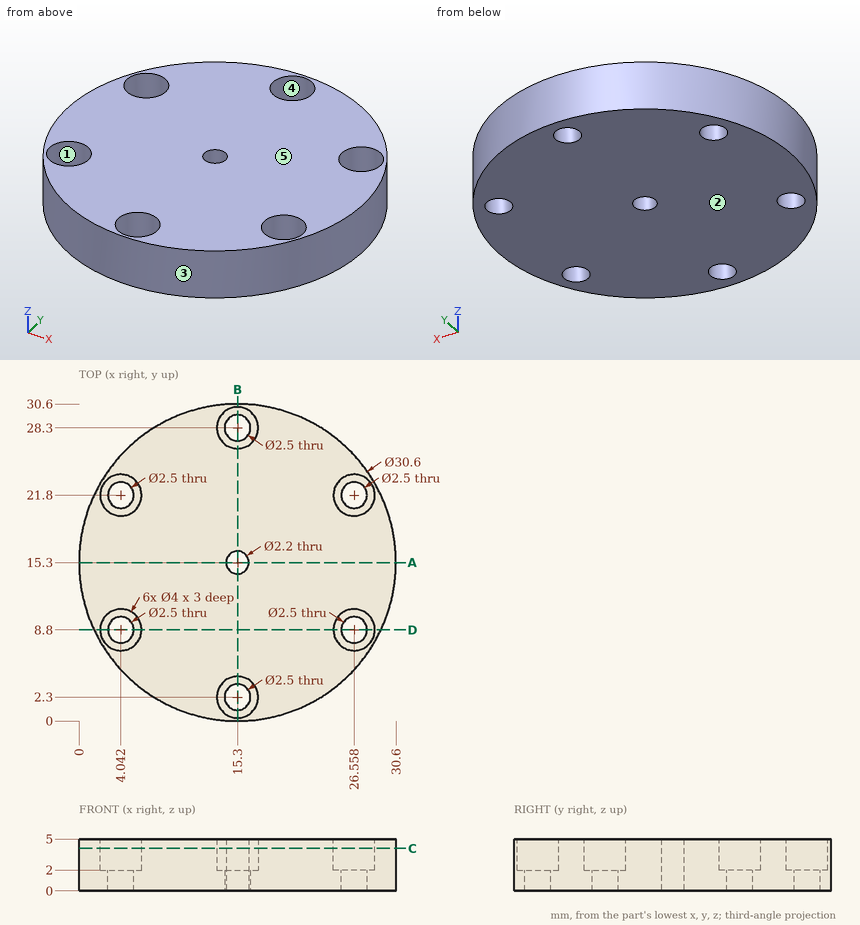
Part print with two shaded views. Sizes in mm from the minimum x, y, z corner. A direction names the side the tool comes from. Round coordinates to 2 decimals unless told otherwise and drop trailing zeros. Loops run counter-clockwise (first coordinate to the right, second up) from the corner with the lowest first, then second, coordinate; pieces in that order, holes last.
Item 1: Saw through at B-B (x = 15.3). List the corners of the cut face in (y, z).
Item 2: Saw through at A-A (y = 15.3). List the corners of the cut face in (x, z), then the cut area to 3 significant figures.
Item 3: Pin check, flat tips, straight feed: P1, Ø2, axis at x = 12, z = 2, coming from the +Y side; P2, Ø2, axis at x = 18, z = 1, coming from the +Y side (1 decimal); P3, Ø3, axis at x = 26.56, y = 8.8, coming from the +Z side. Stop position of each tip, or through.
Item 4: Which spindle directions (+Z, -Z, +X, -X, +Y, -Y) get a long thin tool onto all of the face, cutting with end or side? Do the marked faces 4 and 5. Say none if no direction does.
Item 5: Saw through at C-C (z = 4.1). List the corners of the cut face in (x, y), then the cut area to 3 significant figures.
Item 6: Drill centre lines: line 1 along Y through (x, z) = (15.3, 2.9); line 2 along Y through (x, z) = (15.3, 0.65); line 3 along X through (y, z) = (9.5, 1.15) (1 decimal). Where is each one in solid material? Low to high.
Item 7: Two-plate mould, pull along Y, no slides. Class the marked faces 1, 2 and 3: released by +Y, released by -Y, zero draft, split by the parting line, or undercut.
Item 8: Saw through at D-D (y = 8.8). List the corners of the cut face in (x, z).
Worked answers:
1. outline: (0, 0) - (1.05, 0) - (1.05, 2) - (0.3, 2) - (0.3, 5) - (0, 5) - close; (3.55, 0) - (14.2, 0) - (14.2, 5) - (4.3, 5) - (4.3, 2) - (3.55, 2) - close; (16.4, 0) - (27.05, 0) - (27.05, 2) - (26.3, 2) - (26.3, 5) - (16.4, 5) - close; (29.55, 0) - (30.6, 0) - (30.6, 5) - (30.3, 5) - (30.3, 2) - (29.55, 2) - close
2. outline: (0, 0) - (14.2, 0) - (14.2, 5) - (0, 5) - close; (16.4, 0) - (30.6, 0) - (30.6, 5) - (16.4, 5) - close
2. area: 142 mm2
3. P1: stops at y = 30.43
3. P2: stops at y = 30.5
3. P3: stops at z = 2
4. face 4: +Z
4. face 5: +Z, +X, -X, +Y, -Y
5. outline: circle Ø30.6 at (15.3, 15.3); hole circle Ø4 at (4.04, 8.8); hole circle Ø4 at (4.04, 21.8); hole circle Ø4 at (15.3, 2.3); hole circle Ø4 at (15.3, 28.3); hole circle Ø2.2 at (15.3, 15.3); hole circle Ø4 at (26.56, 8.8); hole circle Ø4 at (26.56, 21.8)
5. area: 656 mm2
6. line 1: y = 0 to 0.3, 4.3 to 14.2, 16.4 to 26.3, 30.3 to 30.6
6. line 2: y = 0 to 1.05, 3.55 to 14.2, 16.4 to 27.05, 29.55 to 30.6
6. line 3: x = 1.1 to 3, 5.1 to 25.5, 27.6 to 29.5
7. face 1: undercut
7. face 2: zero draft
7. face 3: split by the parting line
8. outline: (1.45, 0) - (2.79, 0) - (2.79, 2) - (2.04, 2) - (2.04, 5) - (1.45, 5) - close; (5.29, 0) - (25.31, 0) - (25.31, 2) - (24.56, 2) - (24.56, 5) - (6.04, 5) - (6.04, 2) - (5.29, 2) - close; (27.81, 0) - (29.15, 0) - (29.15, 5) - (28.56, 5) - (28.56, 2) - (27.81, 2) - close
